from build123d import *

# Parameters (mm, degrees)
CROQUIS1_R              = 4
SALIENTE_EXTRUIR1_DEPTH = 3
CROQUIS2_R              = 2.85
SALIENTE_EXTRUIR2_DEPTH = 2
CROQUIS3_R              = 1.125
CORTAR_EXTRUIR1_DEPTH   = 8.549834435
CROQUIS4_R              = 1.875
CORTAR_EXTRUIR2_DEPTH   = 1.5


with BuildPart() as part:
    # Croquis1 → Saliente-Extruir1 (new body)
    with BuildSketch(Plane(origin=(0, 0, 0), x_dir=(1, 0, 0), z_dir=(0, 1, 0))):
        with Locations(Location((0, 0, 0), (0, 0, 270))):
            Circle(CROQUIS1_R)
    extrude(amount=SALIENTE_EXTRUIR1_DEPTH)

    # Croquis2 → Saliente-Extruir2 (add)
    with BuildSketch(Plane(origin=(0, 3, 0), x_dir=(1, 0, 0), z_dir=(0, 1, 0))):
        with Locations(Location((0, 0, 0), (0, 0, 270))):
            Circle(CROQUIS2_R)
    extrude(amount=SALIENTE_EXTRUIR2_DEPTH)

    # Croquis3 → Cortar-Extruir1 (cut, through all)
    with BuildSketch(Plane(origin=(0, 5, 0), x_dir=(1, 0, 0), z_dir=(0, 1, 0))):
        with Locations(Location((0, 0, 0), (0, 0, 270))):
            Circle(CROQUIS3_R)
    extrude(amount=-CORTAR_EXTRUIR1_DEPTH, mode=Mode.SUBTRACT)

    # Croquis4 → Cortar-Extruir2 (cut)
    with BuildSketch(Plane(origin=(0, 5, 0), x_dir=(1, 0, 0), z_dir=(0, 1, 0))):
        with Locations(Location((0, 0, 0), (0, 0, 270))):
            Circle(CROQUIS4_R)
    extrude(amount=-CORTAR_EXTRUIR2_DEPTH, mode=Mode.SUBTRACT)


solid = part.part
The listing builds one solid part. Answer for the finished solid, in the listing's coordinates (mm). A direction names the side the tool comes from. Coordinates: 2 decimals unless noted, no trailing zeros. Order: outer loops, then holes, each group sorted by start corner. A loop starts at its lowest first (then second) coordinate and runs counter-clockwise, first axis right, second up. Notation, with made-up numbers: (8, 7.5) -> (57, 7.5) arc R29 ccw to (57, 30.5) -> close; hole circle Ø5 at (43.25, -40). An arc over 180 degrees is marked (long way). Answer in a Markdown table with one row per item. Add a question column.
Item 1: Find section A-A (x = 0). Write down the section's boundary in (y, z) (3 decimals).
Item 2: Find section D-D (x = -1.5). Write down the section's boundary in (y, z) (3 decimals).
Item 3: Determine the mould class of faces 1 (the face through (-1.734, 3.986, -2.262)), 2 (the face through (0.082, 4.26, -1.873)), 3 (the face through (-1, 3.5, 1)), 4 (the face through (-1, 0, 1)) for opening direction X: +X half, -X half, draft (parallel to the pull), parting line (faces both ways), or undercut.
Item 4: Find section B-B (z = 0). Write down the section's boundary in (x, y) (3 decimals), then the cut area to 3 significant figures.
Item 5: Which of the six approach directions +Z, -Z, +X, -X, +Y, -Y give full straight-line access (tool end or side, diameter ignored) to faces 5 (the face through (0.338, 1.774, 1.073)), 6 (the face through (3, 3, -1))?
Item 6: Each of these flat-tipped pins is pushed along its axis until it touches: P1, Ø2, axis at x = -3, z = -2.5, coming from the +Y side; P2, Ø3.5, axis at x = 0, z = 0, coming from the +Y side; P3, Ø1.5, axis at x = 1.5, z = 0, coming from the +Y side. Where does it stop, or does it pass through?
Item 7: Find the intervals of material crossed by L1, parallel to X at y = 2.7, z = 0 (3 decimals); L2, parallel to X at y = 4.3, z = 0 (3 decimals); L3, parallel to Y at x = -1.5, z = -3, in increasing order. Write a range as from..to.
Item 8: Find section C-C (y = 3.6). Write down the section's boundary in (x, z) (3 decimals), then the cut area to 3 significant figures.
Result set:
| question | item | result |
|---|---|---|
| 1 | outline | (0, -4) -> (3, -4) -> (3, -2.85) -> (5, -2.85) -> (5, -1.875) -> (3.5, -1.875) -> (3.5, -1.125) -> (0, -1.125) -> close; (0, 1.125) -> (3.5, 1.125) -> (3.5, 1.875) -> (5, 1.875) -> (5, 2.85) -> (3, 2.85) -> (3, 4) -> (0, 4) -> close |
| 2 | outline | (0, -3.708) -> (3, -3.708) -> (3, -2.423) -> (5, -2.423) -> (5, -1.125) -> (3.5, -1.125) -> (3.5, 1.125) -> (5, 1.125) -> (5, 2.423) -> (3, 2.423) -> (3, 3.708) -> (0, 3.708) -> close |
| 3 | face 1 | parting line |
| 3 | face 2 | undercut |
| 3 | face 3 | undercut |
| 3 | face 4 | draft |
| 4 | outline | (-4, 0) -> (-1.125, 0) -> (-1.125, 3.5) -> (-1.875, 3.5) -> (-1.875, 5) -> (-2.85, 5) -> (-2.85, 3) -> (-4, 3) -> close; (1.125, 0) -> (4, 0) -> (4, 3) -> (2.85, 3) -> (2.85, 5) -> (1.875, 5) -> (1.875, 3.5) -> (1.125, 3.5) -> close |
| 4 | area | 21.9 mm² |
| 5 | face 5 | +Y, -Y |
| 5 | face 6 | +Y |
| 6 | P1 | stops at y = 3 |
| 6 | P2 | stops at y = 3.5 |
| 6 | P3 | stops at y = 5 |
| 7 | L1 | x = -4..-1.125, 1.125..4 |
| 7 | L2 | x = -2.85..-1.875, 1.875..2.85 |
| 7 | L3 | y = 0..3 |
| 8 | outline | circle Ø5.7 at (0, 0); hole circle Ø3.75 at (0, 0) |
| 8 | area | 14.5 mm² |
